```python
from build123d import *

# Parameters (mm, degrees)
SCHIZZO1_W                    = 64.6
SCHIZZO1_H                    = 20
ESTRUSIONE_ESTRUSIONE1_DEPTH  = 8.2
SCHIZZO2_W                    = 8.2
SCHIZZO2_H                    = 20
ESTRUSIONE_ESTRUSIONE2_DEPTH  = 27.8
SCHIZZO3_W                    = 8.2
SCHIZZO3_H                    = 20
ESTRUSIONE_ESTRUSIONE3_DEPTH  = 27.8
SCHIZZO4_W                    = 8.2
SCHIZZO4_H                    = 20
ESTRUSIONE_ESTRUSIONE4_DEPTH  = 8.2
SCHIZZO5_W                    = 36
SCHIZZO5_H                    = 20
ESTRUSIONE_ESTRUSIONE5_DEPTH  = 8.2
SCHIZZO6_W                    = 48.2
SCHIZZO6_H                    = 19.6
TAGLIO_ESTRUSIONE1_DEPTH      = 77.610443152
F_4_0_4_DIAMETER_HOLE2_D      = 4
F_4_0_4_DIAMETER_HOLE2_DEPTH  = 8.2
RACCORDO3_R                   = 6
SCHIZZO15_W                   = 8.2
SCHIZZO15_H                   = 36
ESTRUSIONE_ESTRUSIONE7_DEPTH  = 3.5
SCHIZZO16_W                   = 8.2
SCHIZZO16_H                   = 36
ESTRUSIONE_ESTRUSIONE8_DEPTH  = 3.5
SCHIZZO17_W                   = 36
SCHIZZO17_H                   = 6
ESTRUSIONE_ESTRUSIONE9_DEPTH  = 11
RACCORDO6_R                   = 2
ESTRUSIONE_ESTRUSIONE11_DEPTH = 58.5
F_4_0_4_DIAMETER_HOLE1_D      = 4
SKETCH1_W                     = 47.8
SKETCH1_H                     = 27
CUT_EXTRUDE1_DEPTH            = 11
SKETCH3_W                     = 10
SKETCH3_H                     = 27
BOSS_EXTRUDE1_DEPTH           = 11
CHAMFER1_SIZE                 = 11
CHAMFER1_SIZE_2               = 38.5


with BuildPart() as part:
    # Schizzo1 → Estrusione-Estrusione1 (new body)
    with BuildSketch(Plane.XY):
        with Locations((32.3, 10)):
            Rectangle(SCHIZZO1_W, SCHIZZO1_H)
    extrude(amount=ESTRUSIONE_ESTRUSIONE1_DEPTH)

    # Schizzo2 → Estrusione-Estrusione2 (add)
    with BuildSketch(Plane.XY.offset(8.2)):
        with Locations((4.1, 10)):
            Rectangle(SCHIZZO2_W, SCHIZZO2_H)
    extrude(amount=ESTRUSIONE_ESTRUSIONE2_DEPTH)

    # Schizzo3 → Estrusione-Estrusione3 (add)
    with BuildSketch(Plane.XY.offset(8.2)):
        with Locations((60.5, 10)):
            Rectangle(SCHIZZO3_W, SCHIZZO3_H)
    extrude(amount=ESTRUSIONE_ESTRUSIONE3_DEPTH)

    # Schizzo4 → Estrusione-Estrusione4 (add)
    with BuildSketch(Plane.ZY.offset(-56.4)):
        with Locations((31.9, 10)):
            Rectangle(SCHIZZO4_W, SCHIZZO4_H)
    extrude(amount=ESTRUSIONE_ESTRUSIONE4_DEPTH)

    # Schizzo5 → Estrusione-Estrusione5 (add)
    with BuildSketch(Plane.ZY):
        with Locations((18, 10)):
            Rectangle(SCHIZZO5_W, SCHIZZO5_H)
    extrude(amount=ESTRUSIONE_ESTRUSIONE5_DEPTH)

    # Schizzo6 → Taglio-Estrusione1 (cut, through all)
    with BuildSketch(Plane.XZ):
        with Locations((24.1, 18)):
            Rectangle(SCHIZZO6_W, SCHIZZO6_H)
    extrude(amount=-TAGLIO_ESTRUSIONE1_DEPTH, mode=Mode.SUBTRACT)

    # Ø4.0 (4) Diameter Hole2
    with Locations(Plane.XY.offset(36)):
        with Locations((52.95, 5), (3.45, 5), (3.45, 15), (52.95, 15)):
            Hole(F_4_0_4_DIAMETER_HOLE2_D / 2, depth=F_4_0_4_DIAMETER_HOLE2_DEPTH)

    # Raccordo3
    raccordo3_edges = [part.edges().sort_by_distance(p)[0] for p in [
        (64.6, 10, 36),
        (64.6, 10, 0),
    ]]
    fillet(raccordo3_edges, radius=RACCORDO3_R)

    # Schizzo15 → Estrusione-Estrusione7 (add)
    with BuildSketch(Plane.XZ):
        with Locations((-4.1, 18)):
            Rectangle(SCHIZZO15_W, SCHIZZO15_H)
    extrude(amount=ESTRUSIONE_ESTRUSIONE7_DEPTH)

    # Schizzo16 → Estrusione-Estrusione8 (add)
    with BuildSketch(Plane(origin=(0, 20, 0), x_dir=(1, 0, 0), z_dir=(0, 1, 0))):
        with Locations((-4.1, -18)):
            Rectangle(SCHIZZO16_W, SCHIZZO16_H)
    extrude(amount=ESTRUSIONE_ESTRUSIONE8_DEPTH)

    # Schizzo17 → Estrusione-Estrusione9 (add)
    with BuildSketch(Plane.ZY.offset(8.2)):
        with Locations((18, 20.5)):
            Rectangle(SCHIZZO17_W, SCHIZZO17_H)
        with Locations((18, -0.5)):
            Rectangle(SCHIZZO17_W, SCHIZZO17_H)
    extrude(amount=ESTRUSIONE_ESTRUSIONE9_DEPTH)

    # Raccordo6
    raccordo6_edges = [part.edges().sort_by_distance(p)[0] for p in [
        (0, -3.5, 18),
        (0, 23.5, 18),
    ]]
    fillet(raccordo6_edges, radius=RACCORDO6_R)

    # Schizzo24 → Estrusione-Estrusione11 (add)
    with BuildSketch(Plane.XY.offset(36)):
        with BuildLine():
            Line((-2, 23.5), (-19.2, 23.5))
            Line((-19.2, 23.5), (-19.2, 17.5))
            Line((-19.2, 17.5), (-8.2, 17.5))
            Line((-8.2, 17.5), (-8.2, 2.5))
            Line((-8.2, 2.5), (-19.2, 2.5))
            Line((-19.2, 2.5), (-19.2, -3.5))
            Line((-19.2, -3.5), (-2, -3.5))
            ThreePointArc((-2, -3.5), (-0.585786438, -2.914213562), (0, -1.5))
            Line((0, -1.5), (0, 21.5))
            ThreePointArc((0, 21.5), (-0.585786438, 22.914213562), (-2, 23.5))
        make_face()
    extrude(amount=ESTRUSIONE_ESTRUSIONE11_DEPTH)

    # Ø4.0 (4) Diameter Hole1 (through all)
    with Locations(Plane(origin=(0, -3.5, 0), x_dir=(-1, 0, 0), z_dir=(0, -1, 0))):
        with Locations((13.7, -85.6), (13.7, -57.6)):
            Hole(F_4_0_4_DIAMETER_HOLE1_D / 2)

    # Sketch1 → Cut-Extrude1 (cut)
    with BuildSketch(Plane.ZY.offset(19.2)):
        with Locations((23.9, 10)):
            Rectangle(SKETCH1_W, SKETCH1_H)
    extrude(amount=-CUT_EXTRUDE1_DEPTH, mode=Mode.SUBTRACT)

    # Sketch3 → Boss-Extrude1 (add)
    with BuildSketch(Plane.ZY.offset(8.2)):
        with Locations((42.8, 10)):
            Rectangle(SKETCH3_W, SKETCH3_H)
    extrude(amount=BOSS_EXTRUDE1_DEPTH)

    # Chamfer1
    # the kernel refuses this chamfer: 38.5, 11 mm, written as the material it adds along each edge
    with BuildSketch(Plane(origin=(-8.2, -3.5, 37.8), x_dir=(-0.9917027448815273, 0, 0.1285521909359956), z_dir=(0, 1, 0))) as chamfer1_piece_1_section:
        Polygon((CHAMFER1_SIZE * 0.991702744882, -CHAMFER1_SIZE * 0.128552190936), (-CHAMFER1_SIZE_2 * 0.128552190936, -CHAMFER1_SIZE_2 * 0.991702744882), (0, 0), align=None)
    chamfer1_piece_1 = extrude(amount=27, mode=Mode.PRIVATE)
    chamfer1_piece_1 = split(chamfer1_piece_1, bisect_by=Plane(origin=(-11.867857143, 10, 0), z_dir=(0, 0, 1)), keep=Keep.TOP, mode=Mode.PRIVATE)
    add(chamfer1_piece_1)


solid = part.part
```
Can you work these out from the model? Positions are in its coordinate system, mm. A direction names the side the tool comes from. Give positions to 0.01 mm unless a question says otherwise; leave off trailing zeros. Order: outer loops, then holes, each group sorted by start corner. A loop starts at its lowest first (then second) coordinate and runs counter-clockwise, first axis right, second up. Notation, with made-up numbers: M 27.5,4 L 48.5,4 A35 cw 48.5,39 Z; hole C 74,54.25 d3. An arc over 180 degrees is marked long. Write item = value, one per line. Start each with the question number.
Q1. I need wall thicknesses on probe 1 along X at (y, z) = (-1.6, 85.6); probe 2 along X at (y, z) = (3.5, 11.5); probe 3 along Y at (x, z) = (3.45, 31.75). Which ranges of each line are inside material? Lowest first, please. Write a range as [from, to].
Q2. Will these pins go through, and if not, where does the flat tip stop? pin 1 Ø6 at (x, y) = (21, 11.5) entering from +Z; pin 2 Ø2 at (y, z) = (1, 68.5) entering from +X; pin 3 Ø4 at (x, z) = (3, 30.5) entering from +Y; pin 4 Ø3.5 at (x, z) = (-13.7, 85.6) entering from +Y.
Q3. Suppose I cut it at D-D (z = 54.5). Write out the boundary of the cut face in (x, y).
Q4. We'd pull the mould along X, two halves only. Please class faces 5 (the cylindrical face through (51.042, 5.601, 31.843)), 6 (the flat face through (4, 20, 32)), 7 (the cylindrical face through (62.889, 10.14, 34.196)): pulls with the +X half, pulls with the -X half, needs draft (parallel to the pull), parting line crosses it, or undercut.
Q5. Suppose I cut it at C-C (y = 15). Write out the boundary of the cut face in (x, z), plus the area to 3 significant figures.
Q6. Suppose I cut it at A-A (z = 85.6). Write out the boundary of the cut face in (x, y).
Q7. For faces 1 (the flat face through (8.2, 10, 32)), 2 (the flat face through (-14, 2.5, 71)), 3 (the flat face through (53, 10, 36)), 4 (the cylindrical face through (1.542, 5.601, 31.843)), which set-ups out of +Z, -Z, +X, -X, +Y, -Y let a thin tool reach every point of the face, with its end or its side?
Q8. Suppose I cut it at B-B (x = 3.45). Write out the boundary of the cut face in (y, z).
Check result:
q1.probe_1 = [-19.2, -15.7], [-11.7, 0]
q1.probe_2 = [-11.69, 0], [56.4, 64.6]
q1.probe_3 = [0, 3], [7, 13], [17, 20]
q2.pin_1 = 8.2
q2.pin_2 = 0
q2.pin_3 = 20
q2.pin_4 = through
q3.outline = M -19.2,-3.5 L -2,-3.5 A2 ccw 0,-1.5 L 0,21.5 A2 ccw -2,23.5 L -19.2,23.5 L -19.2,17.5 L -8.2,17.5 L -8.2,2.5 L -19.2,2.5 Z
q4.face_5 = undercut
q4.face_6 = needs draft
q4.face_7 = pulls with the +X half
q5.outline = M -19.2,37.8 L -8.4,0 L 58.6,0 A6 ccw 64.6,6 L 64.6,30 A6 ccw 58.6,36 L 54.95,36 L 54.95,27.8 L 56.4,27.8 L 56.4,8.2 L 0,8.2 L 0,27.8 L 1.45,27.8 L 1.45,36 L 0,36 L 0,94.5 L -8.2,94.5 L -8.2,47.8 L -19.2,47.8 Z; M 5.45,27.8 L 8.2,27.8 L 8.2,36 L 5.45,36 Z; M 48.2,27.8 L 50.95,27.8 L 50.95,36 L 48.2,36 Z
q5.area = 1,910 mm2
q6.outline = M -19.2,-3.5 L -15.7,-3.5 L -15.7,2.5 L -19.2,2.5 Z; M -19.2,17.5 L -15.7,17.5 L -15.7,23.5 L -19.2,23.5 Z; M -11.7,-3.5 L -2,-3.5 A2 ccw 0,-1.5 L 0,21.5 A2 ccw -2,23.5 L -11.7,23.5 L -11.7,17.5 L -8.2,17.5 L -8.2,2.5 L -11.7,2.5 Z
q7.face_1 = +Z, +Y, -Y
q7.face_2 = +Z, -X
q7.face_3 = +Z, +X, +Y, -Y
q7.face_4 = +Z
q8.outline = M 0,0 L 20,0 L 20,8.2 L 0,8.2 Z; M 0,27.8 L 3,27.8 L 3,36 L 0,36 Z; M 7,27.8 L 13,27.8 L 13,36 L 7,36 Z; M 17,27.8 L 20,27.8 L 20,36 L 17,36 Z
